Build history of the part. All positions in model axes, mm. A direction names the side the tool comes from. Round coordinates to 2 decimals unless told otherwise and drop trailing zeros. Loops run counter-clockwise (first coordinate to the right, second up) from the corner with the lowest first, then second, coordinate; pieces in that order, holes last. Notation, with made-up numbers: M 30,-33 L 71,-33 A18 ccw 71,-3 Z; hole C 70,72 d7. An arc over 180 degrees is marked long. One line per item, written item: value.
Autodesk Inventor part; units mm, degrees
ref_plane "YZ Plane" through (0, 0, 0) normal (1, 0, 0) x (0, 1, 0)
ref_plane "XZ Plane" through (0, 0, 0) normal (0, 1, 0) x (-1, 0, 0)
ref_plane "XY Plane" through (0, 0, 0) normal (0, 0, 1) x (1, 0, 0)
sketch "Sketch1" plane through (0, 0, 0) normal (0, 1, 0) x (-1, 0, 0)
  line L0 (0, 0) -> (6, 0)
  line L1 (6, 0) -> (6, -52)
  line L2 (6, -52) -> (0, -52)
  line L3 (0, -52) -> (0, 0)
  line L4 (6, 0) -> (9, 0)
  line L5 (9, 0) -> (9, -2)
  line L6 (9, -2) -> (6, -2)
  line L7 (6, -2) -> (6, 0)
  line L8 (6, -52) -> (9, -52)
  line L9 (9, -52) -> (9, -50)
  line L10 (9, -50) -> (6, -50)
  line L11 (6, -50) -> (6, -52)
  line L12 (0, 0) -> (4, 0)
  line L13 (4, 0) -> (4, -12)
  line L14 (4, -12) -> (0, -12)
  line L15 (0, -12) -> (0, 0)
  line L16 (0, -52) -> (4, -52)
  line L17 (4, -52) -> (4, -40)
  line L18 (4, -40) -> (0, -40)
  line L19 (0, -40) -> (0, -52)
  line L20 (0, -26) -> (3, -26)
  line L21 (3, -26) -> (3, -34.7)
  line L22 (3, -34.7) -> (3, -17.3)
  circle A0 centre (3, -17.3) radius 1.5
  circle A1 centre (3, -34.7) radius 1.5
  point P0 (0, -40)
  point P1 (6, -50)
  point P2 (6, -2)
  dimension "d0" = 6
  dimension "d1" = 52
  dimension "d2" = 3
  dimension "d3" = 2
  dimension "d4" = 3
  dimension "d5" = 2
  dimension "d6" = 4
  dimension "d7" = 12
  dimension "d8" = 4
  dimension "d9" = 12
  dimension "d10" = 3
  dimension "d11" = 8.7
  dimension "d12" = 17.4
  dimension "d13" = 3
  dimension "d14" = 3
extrude "Extrusion1" add sketch "Sketch1" along normal blind 2 contours L0 L1 L2 L17 L18 L3 L14 L13 | L4 L5 L6 L1 | L10 L9 L8 L1
sketch "Sketch2" plane through (0, 2, 0) normal (0, 1, 0) x (1, 0, 0)
  line L0 (0, 12) -> (0, 40)
  line L1 (0, 26) -> (-6, 26)
  line L2 (-6, 50) -> (-6, 2)
  line L3 (0, 25) -> (-6, 25)
  line L4 (-6, 25) -> (-6, 27)
  line L5 (-6, 27) -> (0, 27)
  line L6 (0, 27) -> (0, 25)
  line L7 (0, 25) -> (-6, 27) construction
  line L8 (-6, 25) -> (0, 27) construction
  point P0 (0, 0)
  point P1 (-3, 26)
  point P2 (0, 25)
  point P3 (0, 27)
  dimension "d17" = 2
extrude "Extrusion2" add sketch "Sketch2" along normal blind 27
sketch "Sketch3" plane through (-6, 0, -50) normal (-1, 0, 0) x (0, 0, 1)
  line L0 (23, 29) -> (25, 29)
  line L1 (25, 2) -> (25, 29)
  line L2 (23, 29) -> (25, 29)
  line L3 (25, 29) -> (25, 27)
  line L4 (25, 27) -> (23, 27)
  line L5 (23, 27) -> (23, 29)
  point P0 (50, 0)
  dimension "d20" = 2
extrude "Extrusion3" add sketch "Sketch3" along normal blind 4
fillet "Fillet1" radius 2 8 edges at (-3, 2, -25) (-3, 2, -27) (-4, 1, -12) (-4, 1, 0) (-4, 1, -52) (0, 1, -40) (0, 1, -12) (-4, 1, -40)
properties part number "battery_holder_1"
Item 1: Wall check: line 1 along X through (y, z) = (1.1, -34.7); line 2 along Z through (x, y) = (-3.25, 1.75); line 3 along Z through (x, y) = (-3, 0.4). Give the ranges that are in metal, low to high.
Check values:
line 1: x = -6 to -4.5, -1.5 to 0
line 2: z = -40.44 to -36.18, -33.22 to -18.78, -15.82 to -11.56
line 3: z = -40.27 to -36.2, -33.2 to -18.8, -15.8 to -11.73
Item 2: Slice it at D-D, the plane z = -37. Give the cut face in (x, y), and give its area (3 significant figures).
Check values:
outline: M -6,0 L 0,0 L 0,2 L -6,2 Z
area: 12.0 mm2
Item 3: Slice it at A-A, the plane x = -6.75. Give the cut face in (y, z).
Check values:
outline: M 0,-52 L 2,-52 L 2,-50 L 0,-50 Z; M 0,-2 L 2,-2 L 2,0 L 0,0 Z; M 27,-27 L 29,-27 L 29,-25 L 27,-25 Z
Item 4: Slice it at C-C, the plane y = 21.25. Give the cut face in (x, z).
Check values:
outline: M -6,-27 L 0,-27 L 0,-25 L -6,-25 Z
Item 5: Pull direction Z, two halves, no side cores. Call faces 6 (the face through (-8, 1, -2)), 7 (the face through (-4.57, 1.01, -51.4)), 8 (the face through (-3, 2, -38)), 9 (the face through (-2.675, 0.986, -15.836)): pulls with the +Z half, pulls with the -Z half, needs draft (parallel to the pull), parting line crosses it, or undercut.
Check values:
face 6: undercut
face 7: pulls with the -Z half
face 8: needs draft
face 9: undercut
Item 6: Slice it at B-B, the plane z = -17.3. Give the cut face in (x, y), and give its area (3 significant figures).
Check values:
outline: M -6,0 L -4.5,0 L -4.5,2 L -6,2 Z; M -1.5,0 L 0,0 L 0,2 L -1.5,2 Z
area: 6.00 mm2
Item 7: Which spindle directions (+Z, -Z, +X, -X, +Y, -Y) get a long thin tool onto all of the face, cutting with end or side? Do faces 1 (the face through (-8, 27, -26)), 2 (the face through (-4, 1, -6)), 3 (the face through (-4, 1, -46)), 4 (the face through (-3, 2, -14)), 5 (the face through (-9, 1, -1)). Say none if no direction does.
Check values:
face 1: +Z, -Z, -X, -Y
face 2: +Z, +X, +Y, -Y
face 3: -Z, +X, +Y, -Y
face 4: +Z, +X, -X, +Y
face 5: +Z, -Z, -X, +Y, -Y
Item 8: Drop flat-ended pins along their axis: P1, Ø2, axis at x = -8, z = -26, coming from the -Y side; P2, Ø3, axis at x = -3, y = 14, coming from the -Z side; P3, Ø3, axis at x = -4.5, y = 21.5, coming from the +Z side. Give the stop position or say it passes through.
Check values:
P1: stops at y = 27
P2: stops at z = -27
P3: stops at z = -25
